Geometry check sheet. Reference: the model listing, model coordinates, mm. A direction names the side the tool comes from. Coordinates: 2 decimals unless noted, no trailing zeros. Loops run counter-clockwise (first coordinate to the right, second up) from the corner with the lowest first, then second, coordinate; pieces in that order, holes last.
from build123d import *

# Parameters (mm, degrees)
BOSS_EXTRUDE1_DEPTH = 12.7
FILLET1_R           = 6.604
FILLET2_R           = 6.604
SKETCH2_R           = 12.7
CUT_EXTRUDE1_DEPTH  = 1173.069644902
CUT_EXTRUDE3_DEPTH  = 1173.069644902
CUT_EXTRUDE4_DEPTH  = 1173.069644902
SKETCH6_R           = 3.3782
CUT_EXTRUDE5_DEPTH  = 1173.069644902
CUT_EXTRUDE6_DEPTH  = 1173.069644902


with BuildPart() as part:
    # Sketch1 → Boss-Extrude1 (new body)
    with BuildSketch(Plane(origin=(0, 0, 0), x_dir=(1, 0, 0), z_dir=(0, 1, 0))):
        Polygon((0, 0), (96.04375, 0), (96.04375, -190.5), (743.74375, -190.5), (743.74375, 0), (838.2, 0), (838.2, 819.15), (0, 819.15), align=None)
        with BuildLine():
            Line((19.05, 41.4782), (31.75, 41.4782))
            ThreePointArc((31.75, 41.4782), (35.1282, 38.1), (31.75, 34.7218))
            Line((31.75, 34.7218), (19.05, 34.7218))
            ThreePointArc((19.05, 34.7218), (15.6718, 38.1), (19.05, 41.4782))
        make_face(mode=Mode.SUBTRACT)
        with BuildLine():
            Line((19.05, 441.5282), (31.75, 441.5282))
            ThreePointArc((31.75, 441.5282), (35.1282, 438.15), (31.75, 434.7718))
            Line((31.75, 434.7718), (19.05, 434.7718))
            ThreePointArc((19.05, 434.7718), (15.6718, 438.15), (19.05, 441.5282))
        make_face(mode=Mode.SUBTRACT)
        with BuildLine():
            Line((31.75, 784.0218), (19.05, 784.0218))
            ThreePointArc((19.05, 784.0218), (15.6718, 787.4), (19.05, 790.7782))
            Line((19.05, 790.7782), (31.75, 790.7782))
            ThreePointArc((31.75, 790.7782), (35.1282, 787.4), (31.75, 784.0218))
        make_face(mode=Mode.SUBTRACT)
        with BuildLine():
            Line((806.45, 784.0218), (819.15, 784.0218))
            ThreePointArc((819.15, 784.0218), (822.5282, 787.4), (819.15, 790.7782))
            Line((819.15, 790.7782), (806.45, 790.7782))
            ThreePointArc((806.45, 790.7782), (803.0718, 787.4), (806.45, 784.0218))
        make_face(mode=Mode.SUBTRACT)
        with BuildLine():
            Line((819.15, 441.5282), (806.45, 441.5282))
            ThreePointArc((806.45, 441.5282), (803.0718, 438.15), (806.45, 434.7718))
            Line((806.45, 434.7718), (819.15, 434.7718))
            ThreePointArc((819.15, 434.7718), (822.5282, 438.15), (819.15, 441.5282))
        make_face(mode=Mode.SUBTRACT)
        with BuildLine():
            Line((819.15, 41.4782), (806.45, 41.4782))
            ThreePointArc((806.45, 41.4782), (803.0718, 38.1), (806.45, 34.7218))
            Line((806.45, 34.7218), (819.15, 34.7218))
            ThreePointArc((819.15, 34.7218), (822.5282, 38.1), (819.15, 41.4782))
        make_face(mode=Mode.SUBTRACT)
    extrude(amount=BOSS_EXTRUDE1_DEPTH)

    # Fillet1
    fillet1_edges = [part.edges().sort_by_distance(p)[0] for p in [
        (743.74375, 6.35, 0),
        (96.04375, 6.35, 0),
    ]]
    fillet(fillet1_edges, radius=FILLET1_R)

    # Fillet2
    fillet2_edges = [part.edges().sort_by_distance(p)[0] for p in [
        (0, 6.35, -819.15),
        (838.2, 6.35, -819.15),
        (838.2, 6.35, 0),
        (743.74375, 6.35, 190.5),
        (96.04375, 6.35, 190.5),
        (0, 6.35, 0),
    ]]
    fillet(fillet2_edges, radius=FILLET2_R)

    # Sketch2 → Cut-Extrude1 (cut, through all)
    with BuildSketch(Plane(origin=(0, 12.7, 0), x_dir=(1, 0, 0), z_dir=(0, 1, 0))):
        with Locations(Location((47.625, 483.87, 0), (0, 0, 270))):
            Circle(SKETCH2_R)
        with Locations(Location((790.575, 483.87, 0), (0, 0, 270))):
            Circle(SKETCH2_R)
    extrude(amount=-CUT_EXTRUDE1_DEPTH, mode=Mode.SUBTRACT)

    # Sketch4 → Cut-Extrude3 (cut, through all)
    with BuildSketch(Plane.XZ):
        with BuildLine():
            Line((350.8375, -527.05), (350.8375, -549.275))
            ThreePointArc((350.8375, -549.275), (327.025, -573.0875), (303.2125, -549.275))
            Line((303.2125, -549.275), (303.2125, -527.05))
            ThreePointArc((303.2125, -527.05), (327.025, -503.2375), (350.8375, -527.05))
        make_face()
        with BuildLine():
            Line((350.8375, 0), (350.8375, -22.225))
            ThreePointArc((350.8375, -22.225), (327.025, -46.0375), (303.2125, -22.225))
            Line((303.2125, -22.225), (303.2125, 0))
            ThreePointArc((303.2125, 0), (327.025, 23.8125), (350.8375, 0))
        make_face()
    extrude(amount=-CUT_EXTRUDE3_DEPTH, mode=Mode.SUBTRACT)

    # Sketch5 → Cut-Extrude4 (cut, through all)
    with BuildSketch(Plane.XZ):
        with BuildLine():
            Line((320.675, -466.725), (320.675, -82.55))
            ThreePointArc((320.675, -82.55), (327.025, -76.2), (333.375, -82.55))
            Line((333.375, -82.55), (333.375, -466.725))
            ThreePointArc((333.375, -466.725), (327.025, -473.075), (320.675, -466.725))
        make_face()
    extrude(amount=-CUT_EXTRUDE4_DEPTH, mode=Mode.SUBTRACT)

    # Sketch6 → Cut-Extrude5 (cut, through all)
    with BuildSketch(Plane.XZ):
        with Locations(Location((354.0125, -274.6375, 0), (0, 0, 270))):
            Circle(SKETCH6_R)
        with Locations(Location((354.0125, -427.0375, 0), (0, 0, 270))):
            Circle(SKETCH6_R)
        with Locations(Location((354.0125, -122.2375, 0), (0, 0, 90))):
            Circle(SKETCH6_R)
        with Locations(Location((300.0375, -427.0375, 0), (0, 0, 90))):
            Circle(SKETCH6_R)
        with Locations(Location((300.0375, -274.6375, 0), (0, 0, 90))):
            Circle(SKETCH6_R)
        with Locations(Location((300.0375, -122.2375, 0), (0, 0, 270))):
            Circle(SKETCH6_R)
    extrude(amount=-CUT_EXTRUDE5_DEPTH, mode=Mode.SUBTRACT)

    # Sketch7 → Cut-Extrude6 (cut, through all)
    with BuildSketch(Plane.XZ):
        with BuildLine():
            ThreePointArc((828.421, -819.15), (833.090733183, -817.215733183), (835.025, -812.546))
            Line((835.025, -812.546), (835.025, -6.604))
            ThreePointArc((835.025, -6.604), (833.090733183, -1.934266817), (828.421, 0))
            Line((828.421, 0), (831.596, 0))
            ThreePointArc((831.596, 0), (836.265733183, -1.934266817), (838.2, -6.604))
            Line((838.2, -6.604), (838.2, -812.546))
            ThreePointArc((838.2, -812.546), (836.265733183, -817.215733183), (831.596, -819.15))
            Line((831.596, -819.15), (828.421, -819.15))
        make_face()
        with BuildLine():
            ThreePointArc((9.525, -812.546), (11.459266817, -817.215733183), (16.129, -819.15))
            Line((16.129, -819.15), (6.604, -819.15))
            ThreePointArc((6.604, -819.15), (1.934266817, -817.215733183), (0, -812.546))
            Line((0, -812.546), (0, -6.604))
            ThreePointArc((0, -6.604), (1.934266817, -1.934266817), (6.604, 0))
            Line((6.604, 0), (16.129, 0))
            ThreePointArc((16.129, 0), (11.459266817, -1.934266817), (9.525, -6.604))
            Line((9.525, -6.604), (9.525, -812.546))
        make_face()
    extrude(amount=-CUT_EXTRUDE6_DEPTH, mode=Mode.SUBTRACT)


solid = part.part
1) Access from +Z, -Z, +X, -X, +Y, -Y to the whole of each face (thin tool, end or side, straight path). Record for faces 1 (the cylindrical face through (327.55, 6.26, -573.08)), 2 (the flat face through (416, 0, -321)).
Data:
face 1: +Y, -Y
face 2: +Z, -Z, +X, -X, -Y
2) Section check A-A on z = -193. Record the cut outline in (x, y) (3 decimals), and give its area (3 significant figures).
Data:
outline: (9.525, 0) - (320.675, 0) - (320.675, 12.7) - (9.525, 12.7) - close; (333.375, 0) - (835.025, 0) - (835.025, 12.7) - (333.375, 12.7) - close
area: 10,300 mm2
3) Mould release check, pull along Z, two halves, no side actions. Record for faces 3 (the flat face through (416, 12.7, -321)), 4 (the cylindrical face through (51.44, 6.439, -471.756)): +Z half, -Z half, draft (parallel to the pull), parting line (faces both ways), or undercut.
Data:
face 3: draft
face 4: undercut
4) Material ranges on probe 1 along X at (y, z) = (8.25, -483.87) (3 decimals); probe 2 along X at (y, z) = (4.5, -483) (3 decimals); probe 3 along X at (y, z) = (3.25, -301) (3 decimals), recorded low to high.
Data:
probe 1: x = 9.525 to 34.925, 60.325 to 777.875, 803.275 to 835.025
probe 2: x = 9.525 to 34.955, 60.295 to 777.905, 803.245 to 835.025
probe 3: x = 9.525 to 320.675, 333.375 to 835.025
5) Depth check by flat-ended pin: pin 1 (6 mm diameter, centred on x = 300.04, z = -122.24, fed in from +Y); pin 2 (4 mm diameter, centred on x = 813, y = 9, fed in from +Z). Enter the tip coordinate at first touch or a pass-through.
Data:
pin 1: passes through
pin 2: stops at z = 0
6) Section check B-B on z = -483.87. Record the cut outline in (x, y) (3 decimals), and give its area (3 significant figures).
Data:
outline: (9.525, 0) - (34.925, 0) - (34.925, 12.7) - (9.525, 12.7) - close; (60.325, 0) - (777.875, 0) - (777.875, 12.7) - (60.325, 12.7) - close; (803.275, 0) - (835.025, 0) - (835.025, 12.7) - (803.275, 12.7) - close
area: 9,840 mm2
7) Section check C-C on y = 5. Count the separate pieces of the cut face and the enclosed holes in it, and give its area (3 significant figures).
Data:
separate pieces: 1
enclosed holes: 17
area: 787,000 mm2
